Model file for the job. Use its own axes, mm. A direction names the side the tool comes from. Coordinates: 2 decimals unless noted, no trailing zeros. Order: outer loops, then holes, each group sorted by start corner. A loop starts at its lowest first (then second) coordinate and runs counter-clockwise, first axis right, second up. Notation, with made-up numbers: (80.5, 33) -> (105.5, 33) arc R31 cw to (105.5, 70) -> close; hole circle Ø4 at (-13, -27.75). An arc over 180 degrees is marked (long way). Return JSON: item names as keys, results as strings. Group by question number.
1) Cut at A-A (z = -45). Write the cut outline in (x, y).
2) Flat gauge pins, fed straight in: pin 1 (2 mm diameter, centred on x = 2, z = -49.5, fed in from +Y); pin 2 (3 mm diameter, centred on x = -4, z = -2, fed in from -Y). Where does each tip first touch, or does it go through?
3) Probe line 1 (Y direction, x = 0, z = 35); line 2 (X direction, y = 0, z = 27.5); line 3 (X direction, y = -0.25, z = -35.5). List the from-to ranges inside material, lowest first.
4) Which spindle directions (+Z, -Z, +X, -X, +Y, -Y) get a long thin tool onto all of the face, cutting with end or side? Do faces 5 (the cylindrical face through (-1.38, 6.2, -67.49)), 6 (the flat face through (6, -3, -63.436)), 7 (the flat face through (6, 3, 63.436)). Say none if no direction does.
5) Pull direction X, two halves, no side cores. Call faces 1 (the flat face through (-3.21, 5.48, -0.89)), 2 (the flat face through (6, 3, -63.436)), 3 (the cylindrical face through (-1.38, -6.2, 67.49)), 4 (the cylindrical face through (-0.767, -2.435, -1)): +X half, -X half, draft (parallel to the pull), parting line (faces both ways), or undercut.
Autodesk Inventor part; units mm, degrees
ref_plane "YZ Plane" through (0, 0, 0) normal (1, 0, 0) x (0, 1, 0)
ref_plane "XZ Plane" through (0, 0, 0) normal (0, 1, 0) x (-1, 0, 0)
ref_plane "XY Plane" through (0, 0, 0) normal (0, 0, 1) x (1, 0, 0)
sketch "Sketch1" plane through (0, 0, 0) normal (0, 0, 1) x (1, 0, 0)
  line L0 (-6.35, -3.6662) -> (-6.35, 3.6662)
  line L1 (-6.35, 3.6662) -> (0, 7.3323)
  line L2 (0, 7.3323) -> (6.35, 3.6662)
  line L3 (6.35, 3.6662) -> (6.35, -3.6662)
  line L4 (6.35, -3.6662) -> (0, -7.3323)
  line L5 (0, -7.3323) -> (-6.35, -3.6662)
  point P0 (0, 0)
  point P1 (0, 0)
  dimension "Size" = 12.7
extrude "Extrusion1" add sketch "Sketch1" along normal mid plane 142.875
sketch "Sketch3" plane through (0, 0, 71.4375) normal (0, 0, 1) x (1, 0, 0)
  line L0 (-6.35, 3.6662) -> (0, 7.3323) construction
  line L1 (0, 7.3323) -> (6.35, 3.6662) construction
  line L2 (6.35, 3.6662) -> (6.35, -3.6662) construction
  line L3 (6.35, -3.6662) -> (0, -7.3323) construction
  line L4 (0, -7.3323) -> (-6.35, -3.6662) construction
  line L5 (-6.35, -3.6662) -> (-6.35, 3.6662) construction
  point P0 (0, 0)
hole "Hole1" at (0, 0, 71.4375) direction (0, 0, -1) diameter 5.1054 end through all
sketch "Sketch4" plane through (0, 0, 71.4375) normal (0, 0, 1) x (1, 0, 0)
  circle A0 centre (0, 0) radius 2.5527 construction
  line L0 (-6.35, 3.6662) -> (0, 7.3323) construction
  line L1 (0, 7.3323) -> (6.35, 3.6662) construction
  line L2 (6.35, 3.6662) -> (6.35, -3.6662) construction
  line L3 (6.35, -3.6662) -> (0, -7.3323) construction
  line L4 (0, -7.3323) -> (-6.35, -3.6662) construction
  line L5 (-6.35, -3.6662) -> (-6.35, 3.6662) construction
  circle A1 centre (0, 0) radius 6.8771
  circle A2 centre (0, 0) radius 8.89
  dimension "thunder" = 13.7541
  dimension "d16" = 17.78
extrude "Extrusion3" cut sketch "Sketch4" against normal through all
sketch "Sketch5" plane through (0, 0, 71.4375) normal (0, 0, 1) x (1, 0, 0)
  arc A0 (5.4616, -4.1791) -> (6.35, -2.6403) centre (0, 0) ccw
  line L0 (5.4616, -4.1791) -> (0.8884, -6.8194)
  arc A1 (-0.8884, -6.8194) -> (0.8884, -6.8194) centre (0, 0) ccw
  line L1 (-0.8884, -6.8194) -> (-5.4616, -4.1791)
  arc A2 (-6.35, -2.6403) -> (-5.4616, -4.1791) centre (0, 0) ccw
  line L2 (-6.35, -2.6403) -> (-6.35, 2.6403)
  arc A3 (-5.4616, 4.1791) -> (-6.35, 2.6403) centre (0, 0) ccw
  line L3 (-5.4616, 4.1791) -> (-0.8884, 6.8194)
  arc A4 (0.8884, 6.8194) -> (-0.8884, 6.8194) centre (0, 0) ccw
  line L4 (0.8884, 6.8194) -> (5.4616, 4.1791)
  arc A5 (6.35, 2.6403) -> (5.4616, 4.1791) centre (0, 0) ccw
  line L5 (6.35, 2.6403) -> (6.35, -2.6403)
  circle A6 centre (0, 0) radius 2.5527
  circle A7 centre (0, 0) radius 6.35
  point P0 (-3.175, 5.4993)
  point P1 (3.175, 5.4993)
  point P2 (6.35, 0)
  point P3 (-6.35, 0)
  point P4 (-3.175, -5.4993)
  point P5 (3.175, -5.4993)
  dimension "d19" = 12.7
extrude "Extrusion4" cut sketch "Sketch5" against normal blind 8.001 contours L0 A7 L5 A0 | L0 A1 L1 A7 | A7 L4 A5 L5 | L1 A2 L2 A7 | A7 L3 A4 L4 | L2 A3 L3 A7
mirror "Mirror2" about plane through (0, 0, 0) normal (0, 0, 1) of "Extrusion4"
equation "\"bearing\" = 25.4"
properties part number "CL4-018" material "Aluminum 6061"
Answers below:
{
 "1": {"outline": "(-6.35, -2.64) arc R6.88 ccw to (-5.46, -4.18) -> (-0.89, -6.82) arc R6.88 ccw to (0.89, -6.82) -> (5.46, -4.18) arc R6.88 ccw to (6.35, -2.64) -> (6.35, 2.64) arc R6.88 ccw to (5.46, 4.18) -> (0.89, 6.82) arc R6.88 ccw to (-0.89, 6.82) -> (-5.46, 4.18) arc R6.88 ccw to (-6.35, 2.64) -> close; hole circle Ø5.11 at (0, 0)"},
 "2": {"pin 1": "stops at y = 6.75", "pin 2": "stops at y = -5.89"},
 "3": {"line 1": "y = -6.88 to -2.55, 2.55 to 6.88", "line 2": "x = -6.35 to -2.55, 2.55 to 6.35", "line 3": "x = -6.35 to -2.54, 2.54 to 6.35"},
 "4": {"face 5": "-Z", "face 6": "-Z, +X, -Y", "face 7": "+Z, +X, +Y"},
 "5": {"face 1": "-X half", "face 2": "draft", "face 3": "parting line", "face 4": "undercut"}
}
